Geometry: final body of the model. Coordinates: model frame, mm. Face numbers are marked on the shaded views. A direction names the side the tool comes from. Give positions to 0.01 mm unless a question says otherwise; leave off trailing zeros. Order: outer loops, then holes, each group sorted by start corner. A loop starts at its lowest first (then second) coordinate and runs counter-clockwise, first axis right, second up. Notation, with made-up numbers: (35.5, 69) - (83.5, 69) arc R20 ccw to (83.5, 107) - close; hole circle Ø4 at (82, 37.5). An arc over 180 degrees is marked (long way). Put each result on its own line as item: value. Start each with the question number.
1. First-contact query: P1, Ø1.5, axis at x = 33, y = -2, coming from the -Z side; P2, Ø4, axis at x = 2.5, z = -8.5, coming from the -Y side; P3, Ø5.5, axis at y = 0, z = 30.5, coming from the +X side. Flat tips, straight axial feed; report the tip coordinate or a pass-through.
2. Mould query, pull axis X, two halves, no side actions, for the marked faces 1, 2 and 3. Classes: pulls with the +X half, pulls with the -X half, needs draft (parallel to the pull), parting line crosses it, or undercut.
3. Section C-C on y = -8.5. Return the cut outline in (x, z).
4. Ray query, line 1 along Y through (x, z) = (21, 36); line 2 along X through (y, z) = (-3, -16.5); line 3 along X through (y, z) = (0.75, 9). Return the intervals inside material, ascending. Write a range as from..to.
5. Section A-A on z = 36. Return the cut outline in (x, y).
6. Set-up query: the marked faces 4, 5, 6 and 7. Return all of +Z, -Z, +X, -X, +Y, -Y with unobstructed straight access to the full face (end or side cutting, diameter ignored); none if empty.
7. Section D-D on x = 36. Return the cut outline in (y, z).
8. Section B-B on z = -15. Return the cut outline in (x, y), plus the area to 3 significant figures.
from build123d import *

# Parameters (mm, degrees)
SKETCH1_W               = 40
SKETCH1_H               = 7
BOSS_EXTRUDE1_DEPTH     = 40
CUT_EXTRUDE1_DEPTH      = 8
FILLET1_R               = 10
SKETCH5_W               = 5
SKETCH5_H               = 7
BOSS_EXTRUDE2_DEPTH     = 20
FILLET2_R               = 7
FILLET3_R               = 3
SKETCH6_R               = 2
CUT_EXTRUDE2_DEPTH      = 41
SKETCH7_R               = 2
CUT_EXTRUDE3_DEPTH      = 23.5
SKETCH8_R               = 6
BOSS_EXTRUDE3_DEPTH     = 40
SKETCH9_W               = 28.10166571
SKETCH9_H               = 14.198736358
CUT_EXTRUDE4_DEPTH      = 4.5000001
CUT_EXTRUDE4_DEPTH_BACK = 10.5000001
SKETCH10_R              = 1.75
CUT_EXTRUDE5_DEPTH      = 41.0000001
FILLET4_R               = 4


with BuildPart() as part:
    # Sketch1 → Boss-Extrude1 (new body)
    with BuildSketch(Plane(origin=(0, 0, 0), x_dir=(0, 0, -1), z_dir=(1, 0, 0))):
        Rectangle(SKETCH1_W, SKETCH1_H)
    extrude(amount=BOSS_EXTRUDE1_DEPTH)

    # Sketch2 → Cut-Extrude1 (cut, through all)
    with BuildSketch(Plane(origin=(0, 3.5, 0), x_dir=(1, 0, 0), z_dir=(0, 1, 0))):
        with BuildLine():
            Line((5, 20), (35, 20))
            Line((35, 20), (35, -5))
            ThreePointArc((35, -5), (32.071067812, -12.071067812), (25, -15))
            Line((25, -15), (15, -15))
            ThreePointArc((15, -15), (7.928932188, -12.071067812), (5, -5))
            Line((5, -5), (5, 20))
        make_face()
    extrude(amount=-CUT_EXTRUDE1_DEPTH, mode=Mode.SUBTRACT)

    # Fillet1
    fillet1_edges = [part.edges().sort_by_distance(p)[0] for p in [
        (40, 0, 20),
        (0, 0, 20),
    ]]
    fillet(fillet1_edges, radius=FILLET1_R)

    # Sketch5 → Boss-Extrude2 (add)
    with BuildSketch(Plane.XY.offset(20)):
        with Locations((20, 0)):
            Rectangle(SKETCH5_W, SKETCH5_H)
    extrude(amount=BOSS_EXTRUDE2_DEPTH)

    # Fillet2
    fillet2_edges = [part.edges().sort_by_distance(p)[0] for p in [
        (17.5, 0, 20),
        (22.5, 0, 20),
    ]]
    fillet(fillet2_edges, radius=FILLET2_R)

    # Fillet3
    fillet3_edges = [part.edges().sort_by_distance(p)[0] for p in [
        (2.5, -3.5, -20),
        (2.5, 3.5, -20),
        (20, -3.5, 40),
        (20, 3.5, 40),
        (37.5, -3.5, -20),
        (37.5, 3.5, -20),
    ]]
    fillet(fillet3_edges, radius=FILLET3_R)

    # Sketch6 → Cut-Extrude2 (cut, through all)
    with BuildSketch(Plane(origin=(40, 0, 0), x_dir=(0, 0, -1), z_dir=(1, 0, 0))):
        with Locations((15, 0)):
            Circle(SKETCH6_R)
    extrude(amount=-CUT_EXTRUDE2_DEPTH, mode=Mode.SUBTRACT)

    # Sketch7 → Cut-Extrude3 (cut, through all)
    with BuildSketch(Plane(origin=(22.5, 0, 0), x_dir=(0, 0, -1), z_dir=(1, 0, 0))):
        with Locations((-36, 0)):
            Circle(SKETCH7_R)
    extrude(amount=-CUT_EXTRUDE3_DEPTH, mode=Mode.SUBTRACT)

    # Sketch8 → Boss-Extrude3 (add)
    with BuildSketch(Plane(origin=(40, 0, 0), x_dir=(0, 0, -1), z_dir=(1, 0, 0))):
        with Locations((-5.366027913, -3.5)):
            Circle(SKETCH8_R)
    extrude(amount=-BOSS_EXTRUDE3_DEPTH)

    # Sketch9 → Cut-Extrude4 (cut, two sides)
    with BuildSketch(Plane(origin=(0, 0, 0), x_dir=(1, 0, 0), z_dir=(0, 1, 0))) as cut_extrude4_sk:
        with Locations((20.049301168, -4.872678537)):
            Rectangle(SKETCH9_W, SKETCH9_H)
    extrude(amount=CUT_EXTRUDE4_DEPTH, mode=Mode.SUBTRACT)
    extrude(cut_extrude4_sk.sketch, amount=-CUT_EXTRUDE4_DEPTH_BACK, mode=Mode.SUBTRACT)

    # Sketch10 → Cut-Extrude5 (cut, through all)
    with BuildSketch(Plane(origin=(40, 0, 0), x_dir=(0, 0, -1), z_dir=(1, 0, 0))):
        with Locations((-5.366027913, -3.5)):
            Circle(SKETCH10_R)
    extrude(amount=-CUT_EXTRUDE5_DEPTH, mode=Mode.SUBTRACT)

    # Fillet4
    fillet4_edges = [part.edges().sort_by_distance(p)[0] for p in [
        (37.5, -3.5, -0.633972087),
        (2.5, -3.5, -0.633972087),
        (3.046104647, -3.5, 11.366027913),
        (37.00319652, -3.5, 11.366027913),
    ]]
    fillet(fillet4_edges, radius=FILLET4_R)


solid = part.part
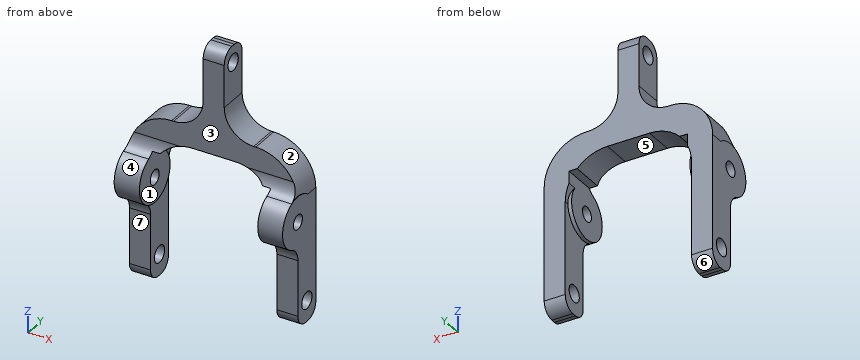
Resolved:
1. P1: z = 11.97
1. P2: y = -3.5
1. P3: x = 22.5
2. face 1: undercut
2. face 2: pulls with the +X half
2. face 3: needs draft
3. outline: (0, 2.05) - (6, 2.05) - (6, 8.68) - (0, 8.68) - close; (34.1, 2.05) - (40, 2.05) - (40, 8.68) - (34.1, 8.68) - close
4. line 1: -3.5..-2, 2..3.5
4. line 2: 0..5, 35..40
4. line 3: 0..6, 34.1..40
5. outline: (17.5, -3.5) - (22.5, -3.5) - (22.5, -2) - (17.5, -2) - close; (17.5, 2) - (22.5, 2) - (22.5, 3.5) - (17.5, 3.5) - close
6. face 4: none
6. face 5: -Z, +Y, -Y
6. face 6: -Z, +X, -X, +Y
6. face 7: -Z, +X, -X, -Y
7. outline: (-5.9, -0.13) arc R4 cw to (-3.5, -3.8) - (-3.5, -17) arc R3 ccw to (-0.5, -20) - (0.5, -20) arc R3 ccw to (3.5, -17) - (3.5, 18) - (-3.5, 18) - (-3.5, 14.53) arc R4 cw to (-5.9, 10.87) arc R6 ccw to start; hole circle Ø3.5 at (-3.5, 5.37); hole circle Ø4 at (0, -15)
8. outline: (0, -3.5) - (5, -3.5) - (5, -2) - (0, -2) - close; (0, 2) - (5, 2) - (5, 3.5) - (0, 3.5) - close; (35, -3.5) - (40, -3.5) - (40, -2) - (35, -2) - close; (35, 2) - (40, 2) - (40, 3.5) - (35, 3.5) - close
8. area: 30.0 mm^2
